Input: part model. Units: mm. Frame: model coordinates. Face numbers are marked on the shaded views. Coordinates: 2 decimals unless noted, no trailing zeros. Write each loop counter-clockwise with the first axis right and the second up, starting at its lowest first coordinate (ties: lowest second). Pieces come first, ordered by that corner, then holes. Notation, with made-up numbers: (74, -31) -> (78, -31) arc R26 ccw to (78, -16) -> close; hole circle Ø9 at (2, 62.25). An arc over 180 degrees is marked (long way). Use one line per item in the form item = value. Start each with the question number.
(1) First-contact query: pin 1 (2 mm diameter, centred on x = 2.5, y = 1, fed in from +Z); pin 2 (4 mm diameter, centred on x = 6.5, z = 3.5, fed in from -Y); pin 3 (3 mm diameter, centred on x = 3.5, y = 1.5, fed in from +Z); pin 4 (6 mm diameter, centred on x = 0, z = 0, fed in from -Y). Flat tips, straight axial feed; report the tip coordinate or a pass-through.
(2) Cut plane B-B on z = 0. Return the cut outline in (x, y), plus the area to 3 significant figures.
(3) Cut plane D-D on y = 1.5. Return the cut outline in (x, z), plus the area to 3 significant figures.
(4) Cut plane A-A on x = 0. Return the cut outline in (y, z), plus the area to 3 significant figures.
(5) Ray query, line 1 along X through (y, z) = (4.5, 0); line 2 along Z through (x, y) = (1.5, 7.5); line 3 along Z through (x, y) = (-3.25, 3). Return the intervals inside material, ascending.
(6) Cut plane C-C on y = 2.5. Return the cut outline in (x, z).
(7) Pull-direction query (X, two-part tool) for the marked faces 1 and 2; classes: released by +X, released by -X, zero draft, split by the parting line, or undercut.
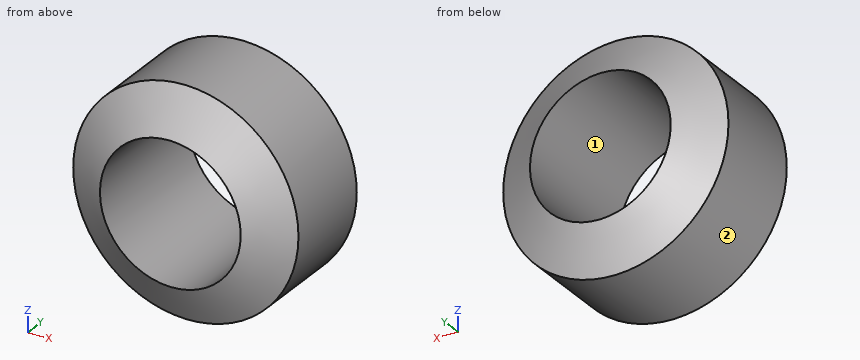
```python
from build123d import *

# Parameters (mm, degrees)
SKETCH2_R           = 8
SKETCH2_R_2         = 5
BOSS_EXTRUDE1_DEPTH = 10
CHAMFER3_SIZE       = 1.75
CHAMFER3_SIZE_2     = 3.031088913
CHAMFER4_SIZE       = 1.75
CHAMFER4_SIZE_2     = 3.031088913


with BuildPart() as part:
    # Sketch2 → Boss-Extrude1 (new body)
    with BuildSketch(Plane(origin=(0, 0, 0), x_dir=(1, 0, 0), z_dir=(0, 1, 0))):
        with Locations(Location((0, 0, 0), (0, 0, 270))):
            Circle(SKETCH2_R)
        with Locations(Location((0, 0, 0), (0, 0, 270))):
            Circle(SKETCH2_R_2, mode=Mode.SUBTRACT)
    extrude(amount=BOSS_EXTRUDE1_DEPTH)

    # Chamfer3
    # the kernel refuses this chamfer: 3.031088913, 1.75 mm, written as the material it takes off along each edge
    with BuildSketch(Plane(origin=(0, 10, 0), x_dir=(0, 0, 1), z_dir=(-1, 0, 0))) as chamfer3_piece_1:
        Polygon((8, -CHAMFER3_SIZE), (8 - CHAMFER3_SIZE_2, 0), (8, 0), align=None)
    revolve(axis=Axis((0, 10, 0), (0, 1, 0)), mode=Mode.SUBTRACT)

    # Chamfer4
    # the kernel refuses this chamfer: 3.031088913, 1.75 mm, written as the material it takes off along each edge
    with BuildSketch(Plane(origin=(0, 0, 0), x_dir=(0, 0, 1), z_dir=(-1, 0, 0))) as chamfer4_piece_1:
        Polygon((8, CHAMFER4_SIZE), (8 - CHAMFER4_SIZE_2, 0), (8, 0), align=None)
    revolve(axis=Axis((0, 0, 0), (0, 1, 0)), mode=Mode.SUBTRACT)


solid = part.part
```
Values:
q1.pin_1 = 7.79
q1.pin_2 = 0.24
q1.pin_3 = 7.74
q1.pin_4 = through
q2.outline = (-8, 1.75) -> (-5, 0.02) -> (-5, 9.98) -> (-8, 8.25) -> close; (5, 0.02) -> (8, 1.75) -> (8, 8.25) -> (5, 9.98) -> close
q2.area = 49.4 mm2
q3.outline = circle Ø15.13 at (0, 0); hole circle Ø10 at (0, 0)
q3.area = 101 mm2
q4.outline = (0.02, -5) -> (1.75, -8) -> (8.25, -8) -> (9.98, -5) -> close; (0.02, 5) -> (9.98, 5) -> (8.25, 8) -> (1.75, 8) -> close
q4.area = 49.4 mm2
q5.line_1 = -8 to -5, 5 to 8
q5.line_2 = -7.86 to -4.77, 4.77 to 7.86
q5.line_3 = -7.31 to -3.8, 3.8 to 7.31
q6.outline = circle Ø16 at (0, 0); hole circle Ø10 at (0, 0)
q7.face_1 = undercut
q7.face_2 = split by the parting line
